CAD build for the part. Positions are in the model's coordinates, mm. A direction names the side the tool comes from. Give positions to 0.01 mm unless a question says otherwise; leave off trailing zeros. Write each loop counter-clockwise with the first axis right and the second up, starting at its lowest first coordinate (ties: lowest second). Pieces come first, ordered by that corner, then holes. Notation, with made-up numbers: (5.5, -34) -> (57.5, -34) arc R28 cw to (57.5, 4) -> close; hole circle Ø7 at (-23, 0.5). An arc over 180 degrees is marked (long way). Answer as a JSON object with one key per item and string values.
```python
from build123d import *

# Parameters (mm, degrees)
F0_R     = 250
F0_R_2   = 125
F1_DEPTH = 827
F2_DEPTH = 57
F3_R     = 15


with BuildPart() as f1:
    # F0 (on Top) → F1 (new body)
    with BuildSketch(Plane.XY):
        Circle(F0_R)
        Circle(F0_R_2, mode=Mode.SUBTRACT)
        Circle(F0_R_2)
    extrude(amount=F1_DEPTH)

    # F0 (on Top) → F2 (join)
    with BuildSketch(Plane.XY):
        Circle(F0_R_2)
    extrude(amount=-F2_DEPTH)

    # F3
    f3_edges = [f1.edges().sort_by_distance(p)[0] for p in [
        (-250, 0, 827),
        (-250, 0, 0),
    ]]
    fillet(f3_edges, radius=F3_R)


solid = f1.part
```
1) Slice it at C-C (z = 449). List the corners of the cut face in (x, y).
Model answer:
{"outline": "circle Ø500 at (0, 0)"}
2) Pin check, flat tips, straight feed: pin 1 (1 mm diameter, centred on x = -4, z = 513.5, fed in from +Y); pin 2 (1.5 mm diameter, centred on y = 138, z = 507.5, fed in from +X); pin 3 (8 mm diameter, centred on x = -143.5, y = 25.5, fed in from -Z). Stop position of each tip, or through.
Model answer:
{"pin 1": "stops at y = 249.98", "pin 2": "stops at x = 208.96", "pin 3": "stops at z = 0"}
3) Slice it at A-A (x = 0). List the corners of the cut face in (y, z).
Model answer:
{"outline": "(-250, 15) arc R15 ccw to (-235, 0) -> (-125, 0) -> (-125, -57) -> (125, -57) -> (125, 0) -> (235, 0) arc R15 ccw to (250, 15) -> (250, 812) arc R15 ccw to (235, 827) -> (-235, 827) arc R15 ccw to (-250, 812) -> close"}
4) Wall check: probe 1 along Z at (x, y) = (117, -115); probe 2 along Y at (x, z) = (-211.5, 412.5); probe 3 along X at (y, z) = (-201, 626). Give the ranges that are in metal, low to high.
Model answer:
{"probe 1": "z = 0 to 827", "probe 2": "y = -133.3 to 133.3", "probe 3": "x = -148.66 to 148.66"}
5) 3-axis set-ups, long thin cutter, end or side, ignore diameter. For faces 1 (the cylindrical face through (-249.76, 10.99, 407.92)), 2 (the flat face through (101, -101, 0)): which of +Z, -Z, +X, -X, +Y, -Y reach the whole face in a straight line?
Model answer:
{"face 1": "+Z, -Z", "face 2": "-Z"}
